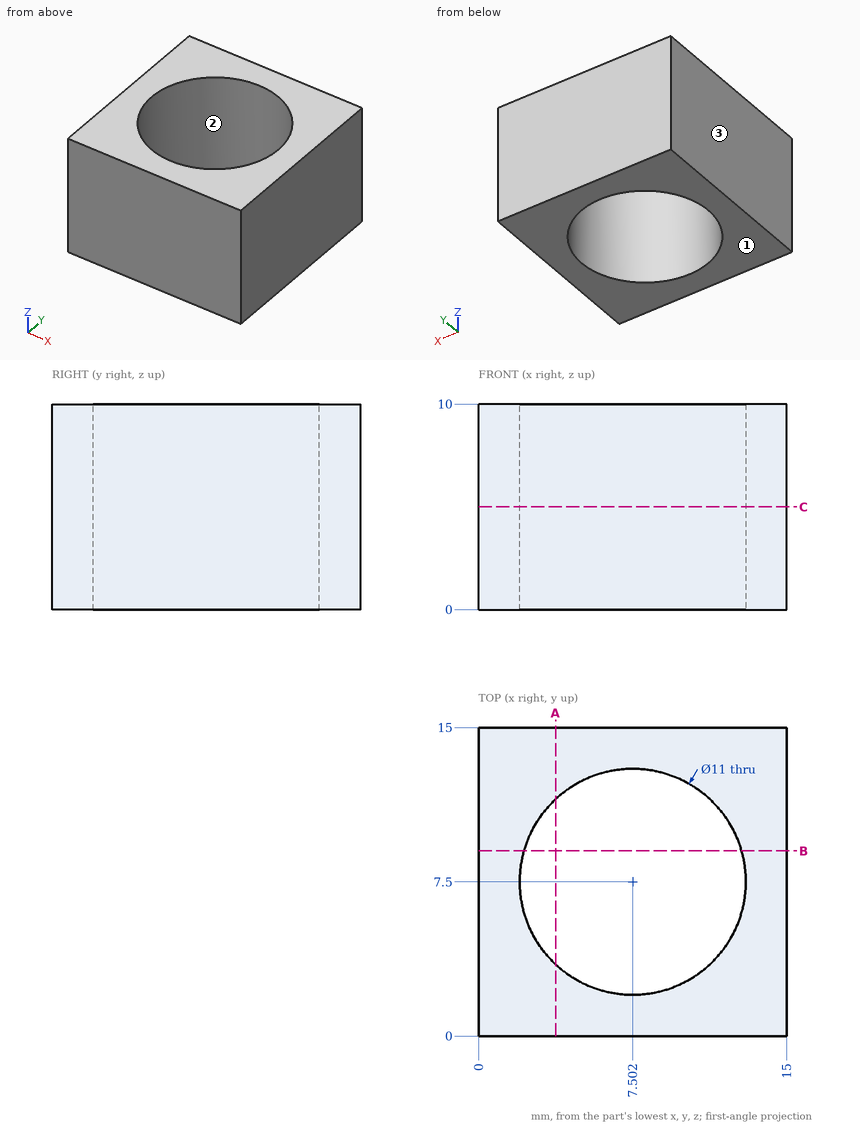
The drawing under review shows one solid part. Ordinate dimensions are in mm from its lowest x, y, z. Round coordinates to 2 decimals unless told otherwise and drop trailing zeros. Order: outer loops, then holes, each group sorted by start corner. A loop starts at its lowest first (then second) coordinate and runs counter-clockwise, first axis right, second up. Notation, with made-up numbers: M -32,66 L 0,66 A14 ccw 0,72 Z; hole C 62,-11.75 d3. An arc over 180 degrees is marked long. Answer as CSV lines item,"result". Start each with the question number.
1) Wall thickness on line 1 along X through (y, z) = (7.5, 3.5); line 2 along Y through (x, z) = (7.75, 5.75); line 3 along X through (y, z) = (2.5, 4.25): over which ranges is each line inside the solid? List them lowest first. Write a range as [from, to].
2) For pin 1 Ø6 at (x, z) = (8, 4) entering from -Y; pin 2 Ø6.5 at (x, y) = (7.5, 7.5) entering from -Z, all flat-tipped, find the tip position at first contact; note any pin that passes through.
3) Add section C-C (z = 5). Give the boundary of the cut face in (x, y).
4) The part is to be moulded in two halves that separate along X. For the marked faces 1, 2 and 3, say which applies: +X half, -X half, draft (parallel to the pull), parting line (faces both ways), or undercut.
5) Add section A-A (x = 3.75). Give the boundary of the cut face in (y, z), then the cut area to 3 significant figures.
6) Add section B-B (y = 9). Give the boundary of the cut face in (x, z).
Resolved:
1,line 1,"[0, 2], [13, 15]"
1,line 2,"[0, 2.01], [12.99, 15]"
1,line 3,"[0, 5.21], [9.79, 15]"
2,pin 1,"y = 0"
2,pin 2,"through"
3,outline,"M 0,0 L 15,0 L 15,15 L 0,15 Z; hole C 7.5,7.5 d11"
4,face 1,"draft"
4,face 2,"undercut"
4,face 3,"-X half"
5,outline,"M 0,0 L 3.48,0 L 3.48,10 L 0,10 Z; M 11.52,0 L 15,0 L 15,10 L 11.52,10 Z"
5,area,"69.6 mm^2"
6,outline,"M 0,0 L 2.21,0 L 2.21,10 L 0,10 Z; M 12.79,0 L 15,0 L 15,10 L 12.79,10 Z"
